```python
from build123d import *

# Parameters (mm, degrees)
CASE_SKETCH_W  = 30
CASE_SKETCH_H  = 57
CASE_SKETCH_R  = 1.35
CASE_2_DEPTH   = 12.8
PORTS_START    = 28.5
PORTS_SKETCH_R = 3.15
PORTS_DEPTH    = 8


with BuildPart() as part:
    # Case Sketch → Case 2 (new body)
    with BuildSketch(Plane(origin=(0, 0, 0), x_dir=(0, 0, -1), z_dir=(1, 0, 0))):
        with Locations((72, 0)):
            Rectangle(CASE_SKETCH_W, CASE_SKETCH_H)
        with Locations((62, -24)):
            Circle(CASE_SKETCH_R, mode=Mode.SUBTRACT)
        with Locations((62, 24)):
            Circle(CASE_SKETCH_R, mode=Mode.SUBTRACT)
        with Locations((81, 0)):
            Circle(CASE_SKETCH_R, mode=Mode.SUBTRACT)
    extrude(amount=-CASE_2_DEPTH)

    # Ports Sketch → Ports (add)
    with BuildSketch(Plane(origin=(0, 0, 0), x_dir=(1, 0, 0), z_dir=(0, 1, 0)).offset(PORTS_START)):
        with Locations(Location((-6.4, 65, 0), (0, 0, 270))):
            Circle(PORTS_SKETCH_R)
        with Locations(Location((-6.4, 79, 0), (0, 0, 270))):
            Circle(PORTS_SKETCH_R)
    extrude(amount=PORTS_DEPTH)


solid = part.part
```
Input: part model. Units: mm. Frame: model coordinates. A direction names the side the tool comes from. Give positions to 0.01 mm unless a question says otherwise; leave off trailing zeros. Loops run counter-clockwise (first coordinate to the right, second up) from the corner with the lowest first, then second, coordinate; pieces in that order, holes last. Notation, with made-up numbers: M 45,56 L 80,56 A19 ccw 80,84 Z; hole C 4.5,75.25 d6. An arc over 180 degrees is marked long. Answer as CSV lines item,"result". Start each with the question number.
1. Section D-D on x = -6.4. Return loops of the section in (y, z), plus the area to 3 significant figures.
2. Section C-C on z = -65. Return loops of the section in (x, y), plus the area to 3 significant figures.
3. Line query: L1, parallel to Y at x = -8.5, z = -62; L2, parallel to Y at x = -6, z = -62; L3, parallel to Y at x = -4.25, z = -81. Output: solid intervals per line, ascending.
4. Section A-A on y = 24. Return loops of the section in (x, z), plus the area to 3 significant figures.
5. Reachability of faces 1 (the face through (-6, 36.5, -65)), 2 (the face through (-6.262, 32.444, -82.147)) from +Z, -Z, +X, -X, +Y, -Y: full face, straight path, thin tool, end or side. Return the list, or none.
6. Pin query (flat end, axial travel): P1, Ø2.5, axis at y = 24, z = -62, coming from the -X side. Return the tip coordinate at first contact, or that it passes through.
7. Section B-B on x = -11.75. Return loops of the section in (y, z), plus the area to 3 significant figures.
Computed values:
1,outline,"M -28.5,-87 L 28.5,-87 L 28.5,-82.15 L 36.5,-82.15 L 36.5,-75.85 L 28.5,-75.85 L 28.5,-68.15 L 36.5,-68.15 L 36.5,-61.85 L 28.5,-61.85 L 28.5,-57 L -28.5,-57 Z; hole C -24,-62 d2.7; hole C 0,-81 d2.7; hole C 24,-62 d2.7"
1,area,"1,790 mm²"
2,outline,"M -12.8,-28.5 L 0,-28.5 L 0,28.5 L -3.25,28.5 L -3.25,36.5 L -9.55,36.5 L -9.55,28.5 L -12.8,28.5 Z"
2,area,"780 mm²"
3,L1,"y = -28.5 to -25.35, -22.65 to 22.65, 25.35 to 28.5"
3,L2,"y = -28.5 to -25.35, -22.65 to 22.65, 25.35 to 36.5"
3,L3,"y = -28.5 to -1.35, 1.35 to 36.5"
4,outline,"M -12.8,-87 L 0,-87 L 0,-63.35 L -12.8,-63.35 Z; M -12.8,-60.65 L 0,-60.65 L 0,-57 L -12.8,-57 Z"
4,area,"349 mm²"
5,face 1,"+Z, -Z, +X, -X, +Y"
5,face 2,"+Y"
6,P1,"passes through"
7,outline,"M -28.5,-87 L 28.5,-87 L 28.5,-57 L -28.5,-57 Z; hole C -24,-62 d2.7; hole C 0,-81 d2.7; hole C 24,-62 d2.7"
7,area,"1,690 mm²"
